The figure shows three views and two pictorial views of one solid part (mm, origin at its lowest corner). Answer the questions. Coordinates: 2 decimals unless noted, no trailing zeros. Loops run counter-clockwise (first coordinate to the right, second up) from the corner with the lowest first, then second, coordinate; pieces in that order, holes last. Notation, with made-up numbers: M 84,13.5 L 134,13.5 A19 ccw 134,17.5 Z; hole C 60,-35 d9. An arc over 180 degrees is marked long. Answer as a JSON object with one key per item and string values. Group by question number.
1. A cutting plane is placed at A-A on y = 15. Give the vertices of the cut face in (x, z), and give its area (3 significant figures).
2. A cutting plane is placed at D-D on z = 12.5. Give the vertices of the cut face in (x, y), and give its area (3 significant figures).
3. Given pin 1 (3 mm diameter, centred on y = 24, z = 3.5, fed in from -X); pin 2 (1 mm diameter, centred on y = 8, z = 25, fed in from -X); pin 3 (1.5 mm diameter, centred on x = 15, y = 15, fed in from +Z), each flat-ended and moving along its own axis, determine where each tip first touches the part or whether it passes through.
4. Straight lines are drawn through the part: L1, parallel to Y at x = 15, z = 8; L2, parallel to Y at x = 14.25, z = 8.75; L3, parallel to X at y = 14.5, z = 23.25. For each, find the intervals that lie inside material, in ascending order.
5. A cutting plane is placed at C-C on z = 20.75. Give the vertices of the cut face in (x, y), and give its area (3 significant figures).
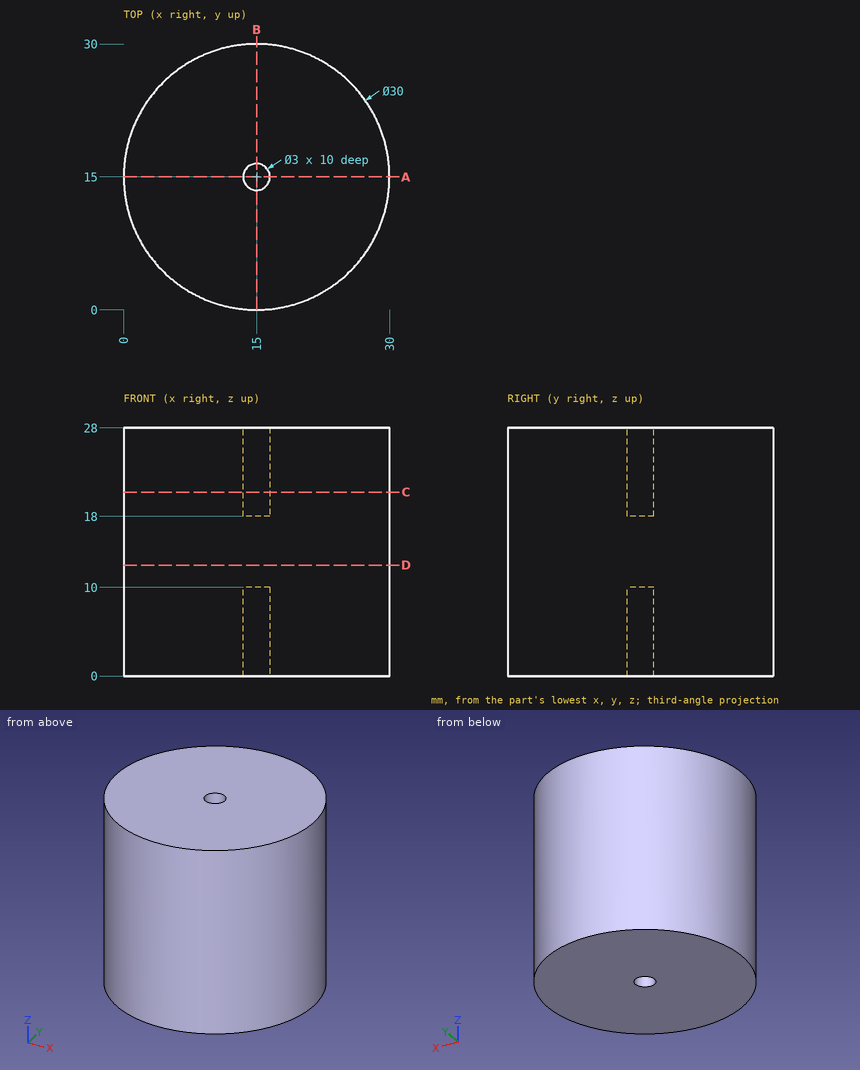
From the geometry:
{
 "1": {"outline": "M 0,0 L 13.5,0 L 13.5,10 L 16.5,10 L 16.5,0 L 30,0 L 30,28 L 16.5,28 L 16.5,18 L 13.5,18 L 13.5,28 L 0,28 Z", "area": "780 mm²"},
 "2": {"outline": "C 15,15 d30", "area": "707 mm²"},
 "3": {"pin 1": "stops at x = 2.01", "pin 2": "stops at x = 1.48", "pin 3": "stops at z = 18"},
 "4": {"L1": "y = 0 to 13.5, 16.5 to 30", "L2": "y = 0.02 to 13.7, 16.3 to 29.98", "L3": "x = 0.01 to 13.59, 16.41 to 29.99"},
 "5": {"outline": "C 15,15 d30; hole C 15,15 d3", "area": "700 mm²"}
}
